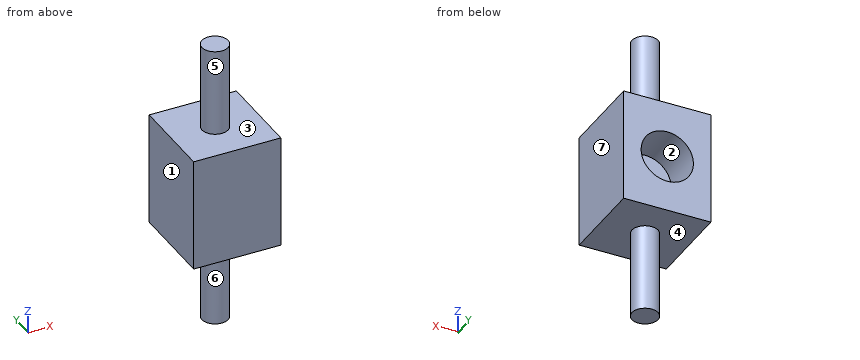
Autodesk Inventor part; units mm, degrees
ref_plane "YZ Plane" through (0, 0, 0) normal (1, 0, 0) x (0, 1, 0)
ref_plane "XZ Plane" through (0, 0, 0) normal (0, 1, 0) x (-1, 0, 0)
ref_plane "XY Plane" through (0, 0, 0) normal (0, 0, 1) x (1, 0, 0)
sketch "Sketch1" plane through (0, 0, 0) normal (0, 0, 1) x (1, 0, 0)
  line L0 (-5, 5) -> (5, 5)
  line L1 (5, 5) -> (5, -5)
  line L2 (5, -5) -> (-5, -5)
  line L3 (-5, -5) -> (-5, 5)
  line L4 (-5, 5) -> (5, -5) construction
  line L5 (5, 5) -> (-5, -5) construction
  point P0 (0, 0)
  dimension "d0" = 10
  dimension "d1" = 10
extrude "Extrusion1" add sketch "Sketch1" along normal blind 13
sketch "Sketch2" plane through (0, 0, 13) normal (0, 0, 1) x (1, 0, 0)
  circle A0 centre (0, 0) radius 1.5
  dimension "d4" = 3
extrude "Extrusion2" add sketch "Sketch2" along normal blind 10
ref_plane "Work Plane1" through (0, 0, 6.5) normal (0, 0, 1) x (1, 0, 0)
mirror "Mirror1" about plane through (0, 0, 6.5) normal (0, 0, 1) of "Extrusion2"
sketch "Sketch3" plane through (-5, 5, 0) normal (0, 1, 0) x (1, 0, 0)
  line L0 (0, 0) -> (0, -13)
  line L1 (0, -6.5) -> (10, -6.5)
  line L2 (10, 0) -> (10, -13)
  circle A0 centre (5, -6.5) radius 3
  point P0 (5, 0)
  dimension "d7" = 6
extrude "Extrusion3" cut sketch "Sketch3" against normal blind 5
properties part number "Claw Connector 1"
The listing builds one solid part. Answer for the finished solid, in the listing's coordinates (mm). Face numbers are marked on the shaded views. A direction names the side the tool comes from. Coordinates: 2 decimals unless noted, no trailing zeros. Loops run counter-clockwise (first coordinate to the right, second up) from the corner with the lowest first, then second, coordinate; pieces in that order, holes last. Notation, with made-up numbers: M 33.5,-21 L 61.5,-21 A23 ccw 61.5,11 Z; hole C 16.25,15.5 d8. An arc over 180 degrees is marked long. Answer as a JSON object with one key per item and string values. Group by question number.
Item 1: Determine the mould class of the marked faces 1, 2, 3 and 4 for opening direction Z: +Z half, -Z half, draft (parallel to the pull), parting line (faces both ways), or undercut.
Item 2: Section B-B (y = 3) is taken. Write down the section's boundary in (x, z).
Item 3: Section C-C (x = 0) is taken. Write down the section's boundary in (y, z), and give its area (3 significant figures).
Item 4: Each of these flat-tipped pins is pushed along its axis until it touches: P1, Ø5, axis at y = -2, z = -3.5, coming from the -X side; P2, Ø5, axis at x = 2.5, y = 1.5, coming from the -Z side; P3, Ø1, axis at x = 3.5, y = 0, coming from the +Z side. Where does it stop, or does it pass through?
Item 5: Which of the six approach directions +Z, -Z, +X, -X, +Y, -Y give full straight-line access (tool end or side, diameter ignored) to the marked faces 5, 6 and 7?
Item 6: Consider L1, parallel to Z at x = 0, y = 3.35; L2, parallel to X at y = 2.75, z = 6.5; L3, parallel to Z at x = 2, y = 3.5. Determine where each line is inside the solid, lowest interval first.
Item 7: Section A-A (z = 6.5) is taken. Write down the section's boundary in (x, y), and give its area (3 significant figures).
Item 8: Section D-D (x = -4) is taken. Write down the section's boundary in (y, z).
Solved:
{
 "1": {"face 1": "draft", "face 2": "undercut", "face 3": "+Z half", "face 4": "-Z half"},
 "2": {"outline": "M -5,0 L 5,0 L 5,13 L -5,13 Z; hole C 0,6.5 d6"},
 "3": {"outline": "M -5,0 L -1.5,0 L -1.5,-10 L 1.5,-10 L 1.5,0 L 5,0 L 5,3.5 L 0,3.5 L 0,9.5 L 5,9.5 L 5,13 L 1.5,13 L 1.5,23 L -1.5,23 L -1.5,13 L -5,13 Z", "area": "160 mm2"},
 "4": {"P1": "stops at x = -1.5", "P2": "stops at z = -10", "P3": "stops at z = 13"},
 "5": {"face 5": "+Z", "face 6": "-Z", "face 7": "+Z, -Z, +X, +Y, -Y"},
 "6": {"L1": "z = 0 to 3.5, 9.5 to 13", "L2": "x = -5 to -3, 3 to 5", "L3": "z = 0 to 4.26, 8.74 to 13"},
 "7": {"outline": "M -5,-5 L 5,-5 L 5,5 L 3,5 L 3,0 L -3,0 L -3,5 L -5,5 Z", "area": "70.0 mm2"},
 "8": {"outline": "M -5,0 L 5,0 L 5,13 L -5,13 Z"}
}
